Work out the finished part from the listing and answer in its coordinate system (mm). A direction names the side the tool comes from. Give positions to 0.01 mm unless a question says otherwise; leave off trailing zeros. Loops run counter-clockwise (first coordinate to the right, second up) from the corner with the lowest first, then second, coordinate; pieces in that order, holes last. Notation, with made-up numbers: M 28,32 L 70,32 A17 ccw 70,64 Z; hole C -34.5,55 d11. An arc over 180 degrees is marked long. Answer as a JSON object with one key per item and string values. Group by question number.
Solid Edge part; units mm, degrees
sketch "Sketch1" plane through (0, 0, 0) normal (1, 0, 0) x (0, 1, 0)
  line L0 (40, 175) -> (-40, 175)
  line L1 (-40, 175) -> (-40, -40)
  line L2 (-40, -40) -> (40, -40)
  line L3 (40, -40) -> (40, 175)
extrude "Protrusion1" add sketch "Sketch1" along normal blind 15
sketch "Sketch2" plane through (0, 0, 35) normal (-1, 0, 0) x (0, -1, 0)
  circle A0 centre (0, -35) radius 18
extrude "Extrusionsausschnitt_1" cut sketch "Sketch2" against normal blind 145
sketch "Sketch3" plane through (0, 0, 35) normal (-1, 0, 0) x (0, -1, 0)
  circle A0 centre (0, -35) radius 21
extrude "Extrusionsausschnitt_2" cut sketch "Sketch3" against normal blind 12
fillet "Verrundung_1" radius 40 2 edges at (7.5, 40, -40) (7.5, -40, -40)
hole "Bohrung_1" at (7.5, -40, 113) direction (0, 1, 0) diameter 4.917 depth 25 tip angle 118 thread major 6 thread length 20
hole "Hole1" at (7.5, -40, 145) direction (0, 1, 0) diameter 4.917 depth 25 tip angle 118 thread major 6 thread length 20
hole "Bohrung_3" at (7.5, 20, 175) direction (0, 0, -1) diameter 4.917 depth 25 tip angle 118 thread major 6 thread length 20
hole "Hole2" at (7.5, -20, 175) direction (0, 0, -1) diameter 4.917 depth 25 tip angle 118 thread major 6 thread length 20
mirror "Mirror1" about plane through (0, 0, 0) normal (0, -1, 0) of "Bohrung_1", "Hole1"
Item 1: For a pull along X with two mould halves and no side action, classify faces 1 (the flat face through (12, -16, 9)), 2 (the cylindrical face through (7.605, -28.595, -27.973)), 3 (the cylindrical face through (8.238, 27.325, 110.655)) as pulls with the +X half, pulls with the -X half, needs draft (parallel to the pull), parting line crosses it, or undercut.
Item 2: A cutting plane is placed at C-C (y = -3.5). Determine the outline of the cut face in (x, z), and give its area (3 significant figures).
Item 3: Find the intervals of material crossed by probe 1 along Y at (x, z) = (7.5, 166); probe 2 along Z at (x, y) = (12.75, 0); probe 3 along X at (y, z) = (20, 155.5), in increasing order. Write a range as [from, to].
Item 4: A cutting plane is placed at D-D (y = 30.5). Determine the outline of the cut face in (x, z).
Item 5: A tool of negligible diameter and unlimited length cuts with its end or side. For faces 4 (the cylindrical face through (5.92, -20.03, 6.31)), 5 (the cylindrical face through (8.44, -27.32, 110.73)), 6 (the flat face through (0, -1, 66)), 7 (the cylindrical face through (8.238, 27.325, 142.655)), from which of +Z, -Z, +X, -X, +Y, -Y can it reach the whole face along a straight path? Write none if from no direction.
Item 6: Given pin 1 Ø4 at (x, y) = (7.5, -20) entering from +Z; pin 2 Ø1 at (x, y) = (6, 24.5) entering from -Z; pin 3 Ø4 at (x, y) = (10.5, 7.5) entering from -Z, each flat-ended and moving along its own axis, determine where each tip first touches the part or whether it passes through.
Item 7: A cutting plane is placed at B-B (z = -5.5). Determine the outline of the cut face in (x, y).
The answers:
{
 "1": {"face 1": "pulls with the -X half", "face 2": "needs draft", "face 3": "undercut"},
 "2": {"outline": "M 0,-39.85 L 15,-39.85 L 15,-17.66 L 12,-17.66 L 12,-20.71 L 0,-20.71 Z; M 0,20.71 L 12,20.71 L 12,17.66 L 15,17.66 L 15,175 L 0,175 Z", "area": "2,620 mm^2"},
 "3": {"probe 1": "y = [-40, -22.46], [-17.54, 17.54], [22.46, 40]", "probe 2": "z = [-40, -18], [18, 175]", "probe 3": "x = [0, 5.04], [9.96, 15]"},
 "4": {"outline": "M 0,-25.88 L 15,-25.88 L 15,175 L 0,175 Z; hole C 7.5,113 d4.92; hole C 7.5,145 d4.92"},
 "5": {"face 4": "-X", "face 5": "-Y", "face 6": "+Z, -Z, -X, +Y, -Y", "face 7": "+Y"},
 "6": {"pin 1": "stops at z = 149.72", "pin 2": "stops at z = -32", "pin 3": "stops at z = -39.62"},
 "7": {"outline": "M 0,-39.62 L 15,-39.62 L 15,-17.14 L 12,-17.14 L 12,-20.27 L 0,-20.27 Z; M 0,20.27 L 12,20.27 L 12,17.14 L 15,17.14 L 15,39.62 L 0,39.62 Z"}
}
